Could you check a few things on this model? Use its own coordinates, in mm. Give positions to 0.01 mm unless a question says otherwise; leave off trailing zeros. Write each loop counter-clockwise with the first axis right and the second up, starting at its lowest first coordinate (ties: lowest second). Pieces come first, ordered by that corner, then holes. Notation, with made-up numbers: (76, 16.25) - (102, 16.25) arc R21 ccw to (102, 44.25) - close; hole circle Ø8 at (31.25, 55.25). An arc over 180 degrees is marked (long way). Answer as CSV lines item,"result". Start each with the question number.
Q1. We'd pull the mould along Z, two halves only. Please class faces 1 (the face through (0, 6, -6)), 2 (the face through (3, 0, 0)), 3 (the face through (0, 6, 6)), 4 (the face through (2.6, 7.94, -0.82)): pulls with the +Z half, pulls with the -Z half, needs draft (parallel to the pull), parting line crosses it, or undercut.
Q2. Imagine slicing it at B-B on x = 0. List the corners of the cut face in (y, z) for me (3 decimals), and give its area (3 significant figures).
Q3. Imagine slicing it at C-C on y = 7.25. List the corners of the cut face in (x, z) for me (3 decimals), and give its area (3 significant figures).
Q4. Imagine slicing it at D-D on y = 1. List the corners of the cut face in (x, z) for me, and give its area (3 significant figures).
Q5. Imagine slicing it at A-A on z = 0. List the corners of the cut face in (x, y) for me (3 decimals), and give its area (3 significant figures).
Q6. If I drill on line 1 along Z through (x, y) = (0, 6.25) (3 decimals); line 2 along Z through (x, y) = (-2.5, 4.25), over which ranges is the centre line in solid material (lowest first)?
Q7. Will this pin go through, and if not, where does the flat tip stop? pin 1 Ø7 at (x, z) = (0, 0) entering from -Y.
```python
from build123d import *

# Parameters (mm, degrees)
SKETCH1_W           = 12
SKETCH1_H           = 12
SKETCH1_R           = 2.725
BOSS_EXTRUDE1_DEPTH = 12
SKETCH2_R           = 2.725
SKETCH2_R_2         = 2.25
BOSS_EXTRUDE2_DEPTH = 4


with BuildPart() as part:
    # Sketch1 → Boss-Extrude1 (new body)
    with BuildSketch(Plane(origin=(0, 0, 0), x_dir=(1, 0, 0), z_dir=(0, 1, 0))):
        Rectangle(SKETCH1_W, SKETCH1_H)
        Circle(SKETCH1_R, mode=Mode.SUBTRACT)
    extrude(amount=BOSS_EXTRUDE1_DEPTH)

    # Sketch2 → Boss-Extrude2 (add)
    with BuildSketch(Plane.XZ):
        Circle(SKETCH2_R)
        Circle(SKETCH2_R_2, mode=Mode.SUBTRACT)
    extrude(amount=-BOSS_EXTRUDE2_DEPTH)


solid = part.part
```
Conclusion:
1,face 1,"pulls with the -Z half"
1,face 2,"needs draft"
1,face 3,"pulls with the +Z half"
1,face 4,"undercut"
2,outline,"(0, -6) - (12, -6) - (12, -2.725) - (4, -2.725) - (4, -2.25) - (0, -2.25) - close; (0, 2.25) - (4, 2.25) - (4, 2.725) - (12, 2.725) - (12, 6) - (0, 6) - close"
2,area,"82.4 mm^2"
3,outline,"(-6, -6) - (6, -6) - (6, 6) - (-6, 6) - close; hole circle Ø5.45 at (0, 0)"
3,area,"121 mm^2"
4,outline,"(-6, -6) - (6, -6) - (6, 6) - (-6, 6) - close; hole circle Ø4.5 at (0, 0)"
4,area,"128 mm^2"
5,outline,"(-6, 0) - (-2.25, 0) - (-2.25, 4) - (-2.725, 4) - (-2.725, 12) - (-6, 12) - close; (2.25, 0) - (6, 0) - (6, 12) - (2.725, 12) - (2.725, 4) - (2.25, 4) - close"
5,area,"82.4 mm^2"
6,line 1,"-6 to -2.725, 2.725 to 6"
6,line 2,"-6 to -1.08, 1.08 to 6"
7,pin 1,"y = 0"
